For this review, take the finished solid that the model builds, in its own axes (mm). A direction names the side the tool comes from. Coordinates: 2 decimals unless noted, no trailing zeros. Loops run counter-clockwise (first coordinate to the right, second up) from the corner with the lowest first, then second, coordinate; pieces in that order, holes last.
```python
from build123d import *

# Parameters (mm, degrees)
CYLINDER1804_R     = 2.5
CYLINDER1804_DEPTH = 30
CYLINDER1805_R     = 2.5
CYLINDER1805_DEPTH = 30
CYLINDER1803_R     = 2.5
CYLINDER1803_DEPTH = 30
CYLINDER1802_R     = 2.5
CYLINDER1802_DEPTH = 30
BOX715_W           = 100
BOX715_H           = 100
BOX715_DEPTH       = 100
TUBE089_R          = 16
TUBE089_R_2        = 12
TUBE089_DEPTH      = 64
CHAMFER060_SIZE    = 2


with BuildPart() as obj1:
    # Cylinder1804 → Cylinder1804 (new body)
    with BuildSketch(Plane(origin=(58, -43, 26), x_dir=(1, 0, 0), z_dir=(0, 0, 1))):
        Circle(CYLINDER1804_R)
    extrude(amount=CYLINDER1804_DEPTH)


with BuildPart() as compound911:
    # Cylinder1805 → Cylinder1805 (new body)
    with BuildSketch(Plane(origin=(58, 11, 26), x_dir=(1, 0, 0), z_dir=(0, 0, 1))):
        Circle(CYLINDER1805_R)
    extrude(amount=CYLINDER1805_DEPTH)

    # Compound911: union obj1
    add(obj1.part)


with BuildPart() as compound911_1:
    # Compound911 placement: moved
    add(compound911.part.moved(Location((34, 0, 13))))


with BuildPart() as obj2:
    # Cylinder1803 → Cylinder1803 (new body)
    with BuildSketch(Plane(origin=(58, -43, 26), x_dir=(1, 0, 0), z_dir=(0, 0, 1))):
        Circle(CYLINDER1803_R)
    extrude(amount=CYLINDER1803_DEPTH)


with BuildPart() as compound912:
    # Cylinder1802 → Cylinder1802 (new body)
    with BuildSketch(Plane(origin=(58, 11, 26), x_dir=(1, 0, 0), z_dir=(0, 0, 1))):
        Circle(CYLINDER1802_R)
    extrude(amount=CYLINDER1802_DEPTH)

    # Compound910: union obj2
    add(obj2.part)


with BuildPart() as compound912_1:
    # Compound910 placement: moved
    add(compound912.part.moved(Location((0, 0, 13))))

    # Compound912: union Compound911
    add(compound911_1.part)


with BuildPart() as krychle715:
    # Box715 → Box715 (new body)
    with BuildSketch(Plane(origin=(32, -54, -63), x_dir=(1, 0, 0), z_dir=(0, 0, 1))):
        with Locations((50, 50)):
            Rectangle(BOX715_W, BOX715_H)
    extrude(amount=BOX715_DEPTH)


with BuildPart() as cut532:
    # Tube089 → Tube089 (new body)
    with BuildSketch(Plane(origin=(75, 16, 42), x_dir=(1, 0, 0), z_dir=(0, -1, 0))):
        Circle(TUBE089_R)
        Circle(TUBE089_R_2, mode=Mode.SUBTRACT)
    extrude(amount=TUBE089_DEPTH)

    # Chamfer060
    chamfer060_edges = [cut532.edges().sort_by_distance(p)[0] for p in [
        (59, -48, 42),
        (59, 16, 42),
    ]]
    chamfer(chamfer060_edges, length=CHAMFER060_SIZE)

    # Cut535: cut Krychle715
    add(krychle715.part, mode=Mode.SUBTRACT)

    # Cut532: cut Compound912
    add(compound912_1.part, mode=Mode.SUBTRACT)


solid = cut532.part
```
Q1. Wall thickness on probe 1 along X at (y, z) = (-14, 42); probe 2 along Y at (x, z) = (60, 42.5); probe 3 along Z at (x, y) = (75, -31.5): over which ranges is each line inside the solid? List them lowest first.
Q2. Consider section A-A (z = 42). State the section outline as (x, y) points, then the cut area to 3 significant figures.
Q3. Consider section C-C (y = -18). State the section outline as (x, z) points.
Q4. For pin 1 Ø8 at (y, z) = (-30, 48) entering from +X; pin 2 Ø1 at (x, y) = (60, 11.5) entering from +Z; pin 3 Ø1 at (x, y) = (90.5, 12) entering from +Z, all flat-tipped, find the tip position at first contact; note any pin that passes through.
Q5. Consider section B-B (x = 75). State the section outline as (y, z) points.
Q6. Machinability: for faces 5 (the face through (74.9, 16, 54.3)), 6 (the face through (90, 11, 39)), 7 (the face through (60.5, 11, 42.7)), which of the approach directions +Z, -Z, +X, -X, +Y, -Y give a long, thin tool a straight path to every point of the face, cutting with its end or side? Answer none if there is none.
Q7. The part is to be moulded in two halves that separate along X. For faces 1 (the face through (75, -16, 58)), 2 (the face through (74.9, -48, 54.3)), 3 (the face through (75, -16, 54)), 4 (the face through (89.5, 11, 42.7)), say which applies: +X half, -X half, draft (parallel to the pull), parting line (faces both ways), or undercut.
Model answer:
1. probe 1: x = 59 to 63, 87 to 91
1. probe 2: y = -46.99 to -44.5, -41.5 to 9.5, 12.5 to 14.99
1. probe 3: z = 54 to 58
2. outline: (59, -46) - (61, -48) - (63, -48) - (63, 16) - (61, 16) - (59, 14) - (59, 13.29) arc R2.5 cw to (59, 8.71) - (59, -40.71) arc R2.5 cw to (59, -45.29) - close; (87, -48) - (89, -48) - (91, -46) - (91, -45.29) arc R2.5 cw to (91, -40.71) - (91, 8.71) arc R2.5 cw to (91, 13.29) - (91, 14) - (89, 16) - (87, 16) - close
2. area: 484 mm2
3. outline: (59.8, 37) - (64.09, 37) arc R12 cw (long way) to (85.91, 37) - (90.2, 37) arc R16 ccw (long way) to start
4. pin 1: stops at x = 90.87
4. pin 2: stops at z = 48.76
4. pin 3: stops at z = 39
5. outline: (-48, 54) - (16, 54) - (16, 56) - (14, 58) - (-46, 58) - (-48, 56) - close
6. face 5: +Z, -Z, +X, -X, +Y
6. face 6: +Z, +X
6. face 7: +Z, -X
7. face 1: parting line
7. face 2: draft
7. face 3: undercut
7. face 4: +X half
